```python
from build123d import *

# Parameters (mm, degrees)
SKETCH1_W           = 309.23
SKETCH1_H           = 88.841000118
BOSS_EXTRUDE1_DEPTH = 3.175
CUT_EXTRUDE2_DEPTH  = 161.90077587


with BuildPart() as part:
    # Sketch1 → Boss-Extrude1 (new body)
    with BuildSketch(Plane.XY):
        Rectangle(SKETCH1_W, SKETCH1_H)
    extrude(amount=BOSS_EXTRUDE1_DEPTH)

    # Sketch4 → Cut-Extrude2 (cut, through all)
    with BuildSketch(Plane.XY.offset(3.175)):
        Polygon((33.965, 6.320500059), (154.615, 6.320500059), (154.615, 44.420500059), (8.565, 44.420500059), (8.565, 29.000644342), align=None)
    extrude(amount=-CUT_EXTRUDE2_DEPTH, mode=Mode.SUBTRACT)


solid = part.part
```
Build history of the part. All positions in model axes, mm. Round coordinates to 2 decimals unless told otherwise and drop trailing zeros. Write each loop counter-clockwise with the first axis right and the second up, starting at its lowest first coordinate (ties: lowest second). Pieces come first, ordered by that corner, then holes.
1) Band-saw the part on A-A, the plane z = 2.15. List the corners of the cut face in (x, y) (1 decimal), and give its area (3 significant figures).
2) Drill centre lines: probe 1 along Y at (x, z) = (116.5, 1.95); probe 2 along X at (y, z) = (36, 2.6) (3 decimals); probe 3 along X at (y, z) = (14, 0.9) (3 decimals). Where is each one in solid material? Low to high.
3) Band-saw the part on B-B, the plane y = 35. List the corners of the cut face in (x, z) (3 decimals).
4) Band-saw the part on C-C, the plane x = 63. List the corners of the cut face in (y, z) (1 decimal), and give its area (3 significant figures).
Ans:
1. outline: (-154.6, -44.4) - (154.6, -44.4) - (154.6, 6.3) - (34, 6.3) - (8.6, 29) - (8.6, 44.4) - (-154.6, 44.4) - close
1. area: 22,200 mm2
2. probe 1: y = -44.42 to 6.32
2. probe 2: x = -154.615 to 8.565
2. probe 3: x = -154.615 to 25.365
3. outline: (-154.615, 0) - (8.565, 0) - (8.565, 3.175) - (-154.615, 3.175) - close
4. outline: (-44.4, 0) - (6.3, 0) - (6.3, 3.2) - (-44.4, 3.2) - close
4. area: 161 mm2
